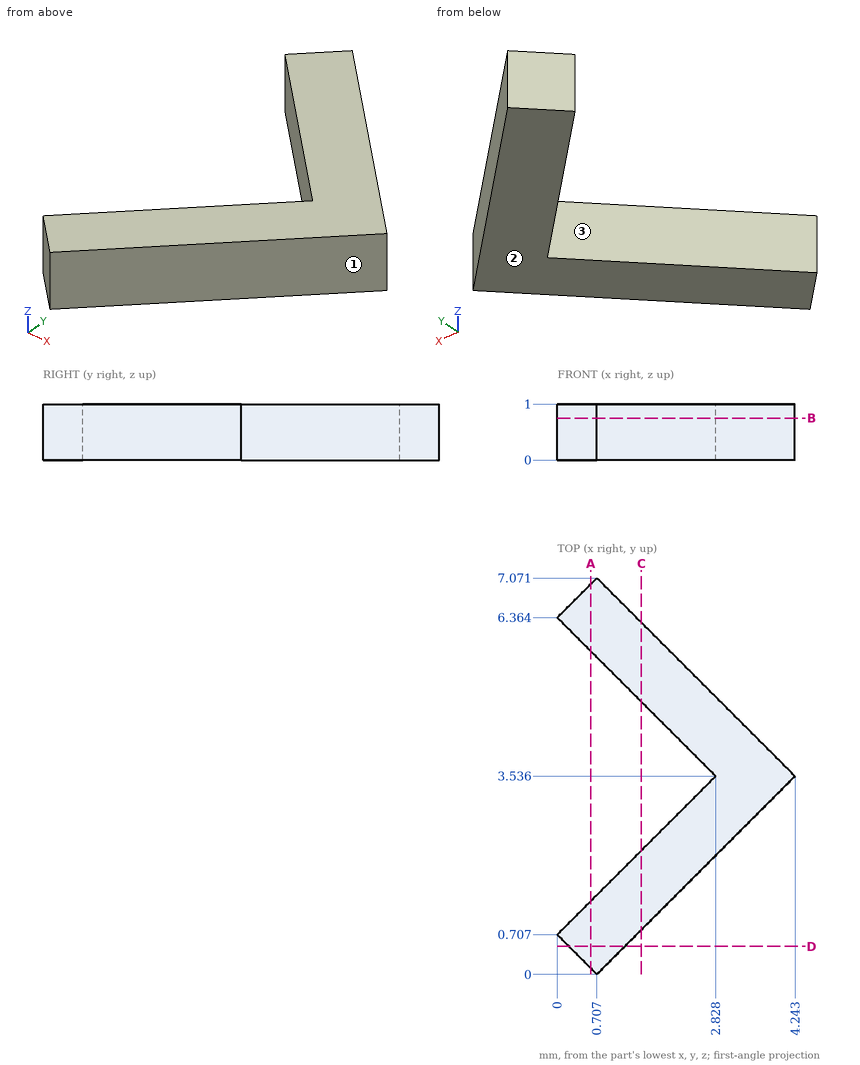
Could you check a few things on this drawing? It's one solid part, dimensions in mm from its lowest x, y, z. Coordinates: 2 decimals unless noted, no trailing zeros. Loops run counter-clockwise (first coordinate to the right, second up) from the corner with the lowest first, then second, coordinate; pieces in that order, holes last. Notation, with made-up numbers: (-16.5, 65.5) - (18.5, 65.5) arc R4 cw to (18.5, 69.5) - close; hole circle Ø3 at (64.25, -23). An arc over 180 degrees is marked (long way). Answer as a JSON object with one key per item and string values. Group by question number.
Item 1: If we section it at A-A (x = 0.6): List the corners of the cut face in (y, z) for me.
Item 2: If I drill on L1, parallel to Y at x = 0.75, z = 0.9 (1 decimal); L2, parallel to Y at x = 2.3, z = 0.5 (1 decimal); L3, parallel to X at y = 6.5, z = 0.8 (1 decimal), over which ranges is the centre line in solid material (lowest first)? Write a range as from..to.
Item 3: If we section it at D-D (y = 0.5): List the corners of the cut face in (x, z) for me.
Item 4: If we section it at C-C (x = 1.5): List the corners of the cut face in (y, z) for me.
Item 5: If we section it at B-B (z = 0.75): List the corners of the cut face in (x, y) for me (1 decimal).
Item 6: If we mould it in two halves opening along Y, with no side actions, what happens to the marked faces 1, 2 and 3? For each: released by +Y, released by -Y, zero draft, split by the parting line, or undercut.
Returned:
{
 "1": {"outline": "(0.11, 0) - (1.31, 0) - (1.31, 1) - (0.11, 1) - close; (5.76, 0) - (6.96, 0) - (6.96, 1) - (5.76, 1) - close"},
 "2": {"L1": "y = 0..1.5, 5.6..7", "L2": "y = 1.6..3, 4.1..5.5", "L3": "x = 0.1..1.3"},
 "3": {"outline": "(0.21, 0) - (1.21, 0) - (1.21, 1) - (0.21, 1) - close"},
 "4": {"outline": "(0.79, 0) - (2.21, 0) - (2.21, 1) - (0.79, 1) - close; (4.86, 0) - (6.28, 0) - (6.28, 1) - (4.86, 1) - close"},
 "5": {"outline": "(0, 0.7) - (0.7, 0) - (4.2, 3.5) - (0.7, 7.1) - (0, 6.4) - (2.8, 3.5) - close"},
 "6": {"face 1": "released by -Y", "face 2": "zero draft", "face 3": "undercut"}
}
